from build123d import *

# Parameters (mm, degrees)
BASE_FLANGE1_DEPTH        = 3.2
SKETCH8_R                 = 1.635
CUT_EXTRUDE1_DEPTH        = 3.2
F_4_CLEARANCE_HOLE2_D     = 3.2639
F_4_CLEARANCE_HOLE2_DEPTH = 3.2
F_4_CLEARANCE_HOLE2_TIP   = 0.980574487
CUT_EXTRUDE2_DEPTH        = 3.2


# Sheet-metal steps are written as plain solids
with BuildPart() as part:
    # Sketch3 → Base-Flange1 (new body)
    with BuildSketch(Plane(origin=(0, 0, 0), x_dir=(1, 0, 0), z_dir=(0, 1, 0))):
        with BuildLine():
            Line((-29.358964924, 8.867320879), (-29.358964924, 25.825))
            Line((-29.358964924, 25.825), (-29.358964924, 48.325))
            Line((-29.358964924, 48.325), (-19.358964924, 48.325))
            Line((-19.358964924, 48.325), (-19.358964924, 25.825))
            Line((-19.358964924, 25.825), (29.358964924, 25.825))
            Line((29.358964924, 25.825), (29.358964924, 8.867320879))
            ThreePointArc((29.358964924, 8.867320879), (23.15, 10.825), (16.941035076, 8.867320879))
            ThreePointArc((16.941035076, 8.867320879), (11.575, 6.362392354), (6.208964924, 8.867320879))
            ThreePointArc((6.208964924, 8.867320879), (0, 10.825), (-6.208964924, 8.867320879))
            ThreePointArc((-6.208964924, 8.867320879), (-11.575, 6.362392354), (-16.941035076, 8.867320879))
            ThreePointArc((-16.941035076, 8.867320879), (-23.15, 10.825), (-29.358964924, 8.867320879))
        make_face()
    extrude(amount=-BASE_FLANGE1_DEPTH)

    # Sketch8 → Cut-Extrude1 (cut)
    with BuildSketch(Plane(origin=(0, 0, 0), x_dir=(1, 0, 0), z_dir=(0, 1, 0))):
        with Locations(Location((-24.358964924, 44.325, 0), (0, 0, 270))):
            Circle(SKETCH8_R)
        with Locations(Location((-24.358964924, 34.825, 0), (0, 0, 270))):
            Circle(SKETCH8_R)
    extrude(amount=-CUT_EXTRUDE1_DEPTH, mode=Mode.SUBTRACT)

    # #4 Clearance Hole2
    with Locations(Plane.XZ.offset(3.2)):
        with Locations((11.575, -18.325), (-11.575, -18.325)):
            Hole(F_4_CLEARANCE_HOLE2_D / 2, depth=F_4_CLEARANCE_HOLE2_DEPTH)
            with Locations((0, 0, -(F_4_CLEARANCE_HOLE2_DEPTH + F_4_CLEARANCE_HOLE2_TIP / 2))):  # 118° drill point
                Cone(0, F_4_CLEARANCE_HOLE2_D / 2, F_4_CLEARANCE_HOLE2_TIP, mode=Mode.SUBTRACT)

    # Sketch11 → Cut-Extrude2 (cut)
    with BuildSketch(Plane.XZ.offset(3.2)):
        with BuildLine():
            Line((-29.645753142, -9.276896902), (-29.645753142, -3.891418545))
            Line((-29.645753142, -3.891418545), (33.433786827, -3.891418545))
            Line((33.433786827, -3.891418545), (33.433786827, -25.825))
            Line((33.433786827, -25.825), (28.858964924, -25.825))
            Line((28.858964924, -25.825), (28.858964924, -9.780764004))
            ThreePointArc((28.858964924, -9.780764004), (22.648874034, -11.313907272), (16.598650974, -9.237718925))
            ThreePointArc((16.598650974, -9.237718925), (11.575, -6.862392354), (6.551349026, -9.237718925))
            ThreePointArc((6.551349026, -9.237718925), (0, -11.325), (-6.551349026, -9.237718925))
            ThreePointArc((-6.551349026, -9.237718925), (-11.575, -6.862392354), (-16.598650974, -9.237718925))
            ThreePointArc((-16.598650974, -9.237718925), (-23.115993323, -11.324948942), (-29.645753142, -9.276896902))
        make_face()
    extrude(amount=-CUT_EXTRUDE2_DEPTH, mode=Mode.SUBTRACT)


solid = part.part
The model under review builds one solid part; all positions refer to its coordinate system, in mm. A direction names the side the tool comes from. Round coordinates to 2 decimals unless told otherwise and drop trailing zeros. Write each loop counter-clockwise with the first axis right and the second up, starting at its lowest first coordinate (ties: lowest second). Pieces come first, ordered by that corner, then holes. Notation, with made-up numbers: (29, -28.75) - (87, -28.75) arc R12 cw to (87, -22.75) - close; hole circle Ø5 at (-36.5, 5.25). An arc over 180 degrees is marked (long way). One line per item, written item: value. Start each with the question number.
1. To check wall thickness, follow L1, parallel to X at y = -0.15, z = -30; L2, parallel to X at y = -0.3, z = -35; L3, parallel to X at y = -2, z = -10. State the ranges of each line that lie inside material, in increasing order. Write a range as from..to.
2. The part is to be moulded in two halves that separate along X. For faces 1 (the face through (-19.359, -2, -37)), 2 (the face through (-12.452, -1.578, -16.949)), 3 (the face through (-24, -2, -48.325)), say which applies: released by +X, released by -X, zero draft, split by the parting line, or undercut.
3. Consider section D-D on x = -3. Write out the cut boundary in (y, z) (3 decimals).
4. Consider section A-A on z = -44. Write out the cut boundary in (x, y), and give its area (3 significant figures).
5. Consider section B-B on y = -1.95. Write out the cut boundary in (x, z) (3 decimals).
6. Consider section C-C on z = -30. Write out the cut boundary in (x, y).
7. Clearance check with flat-ended pins moving along their axes: P1, Ø1.5, axis at x = 15.5, y = -2, coming from the -Z side (3 decimals); P2, Ø1.5, axis at x = 15, y = -3, coming from the +Z side. State where each tip first meets the part, or that it passes through.
8. Machinability: for faces 4 (the face through (4, -2, -25.825)), 5 (the face through (22.74, -1.622, -11.318)), which of the approach directions +Z, -Z, +X, -X, +Y, -Y give a long, thin tool a straight path to every point of the face, cutting with its end or side? Answer none if there is none.
Checks:
1. L1: x = -29.36..-19.36
1. L2: x = -29.36..-25.98, -22.73..-19.36
1. L3: x = -29.36..-28.47, -17.83..-5.32, 5.32..17.83, 28.47..28.86
2. face 1: released by +X
2. face 2: undercut
2. face 3: zero draft
3. outline: (-3.2, -25.825) - (0, -25.825) - (0, -10.92) - (-3.2, -10.92) - close
4. outline: (-29.36, -3.2) - (-25.96, -3.2) - (-25.96, 0) - (-29.36, 0) - close; (-22.76, -3.2) - (-19.36, -3.2) - (-19.36, 0) - (-22.76, 0) - close
4. area: 21.7 mm^2
5. outline: (-29.359, -48.325) - (-19.359, -48.325) - (-19.359, -25.825) - (28.859, -25.825) - (28.859, -9.781) arc R11.325 cw to (16.599, -9.238) arc R6.5 ccw to (6.551, -9.238) arc R11.325 cw to (-6.551, -9.238) arc R6.5 ccw to (-16.599, -9.238) arc R11.325 cw to (-29.359, -9.471) - close; hole circle Ø3.27 at (-24.359, -44.325); hole circle Ø3.27 at (-24.359, -34.825); hole circle Ø3.264 at (-11.575, -18.325); hole circle Ø3.264 at (11.575, -18.325)
6. outline: (-29.36, -3.2) - (-19.36, -3.2) - (-19.36, 0) - (-29.36, 0) - close
7. P1: stops at z = -25.825
7. P2: stops at z = -7.44
8. face 4: -Z, +X, +Y, -Y
8. face 5: +Z, +Y, -Y
